For this review, use the dimensioned drawing (mm, ordinates from the lowest corner) and the shaded views. Give positions to 0.01 mm unless a question says otherwise; leave off trailing zeros.
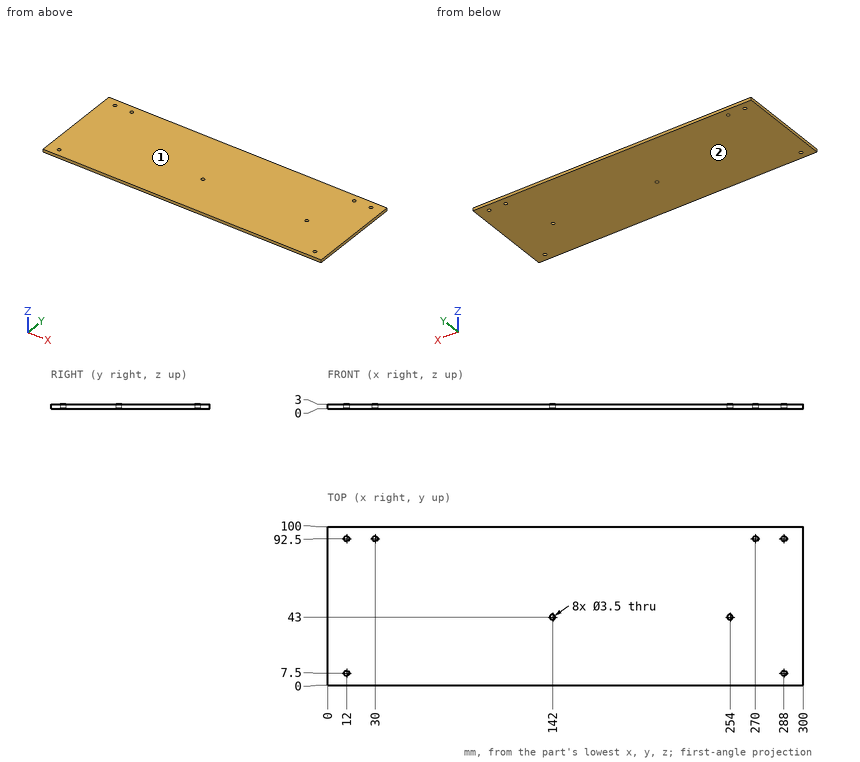
(1) The part is to be moulded in two halves that separate along Z. For the marked faces 1 and 2, say which applies: +Z half, -Z half, draft (parallel to the pull), parting line (faces both ways), or undercut.
(2) For L1, parallel to Y at x = 288, z = 0.65; L2, parallel to X at y = 92.5, z = 1.65; L3, parallel to Y at x = 270, z = 1, list the stretches that pass through material, from the lowest coordinate up.
(3) Clearance check with a flat-ended pin moving along its axis: pin 1 Ø2 at (x, y) = (288, 7.5) entering from +Z. State where the tip first meets the part, or that it passes through.
The answers:
1. face 1: +Z half
1. face 2: -Z half
2. L1: y = 0 to 5.75, 9.25 to 90.75, 94.25 to 100
2. L2: x = 0 to 10.25, 13.75 to 28.25, 31.75 to 268.25, 271.75 to 286.25, 289.75 to 300
2. L3: y = 0 to 90.75, 94.25 to 100
3. pin 1: passes through
